Can you work these out from the model? Positions are in its coordinate system, mm. A direction names the side the tool comes from. Give positions to 0.01 mm unless a question says otherwise; leave off trailing zeros. Write each loop counter-clockwise with the first axis right and the second up, starting at its lowest first coordinate (ties: lowest second). Pieces come first, ordered by that corner, then holes.
from build123d import *

# Parameters (mm, degrees)
SKETCH1_R            = 50
BOSS_EXTRUDE1_DEPTH  = 5
SKETCH2_R            = 25.1
SKETCH2_R_2          = 21.1
SKETCH2_R_3          = 12.4
SKETCH2_R_4          = 9.399999999999999
BOSS_EXTRUDE2_DEPTH  = 5
CHAMFER1_SIZE        = 1
CUT_EXTRUDE1_START   = -5
SKETCH3_R            = 9.399999999999997
CUT_EXTRUDE1_DEPTH   = 5
CUT_EXTRUDE2_DEPTH   = 5
BOSS_EXTRUDE3_DEPTH  = 5
SKETCH6_R            = 1.5000000000000009
SKETCH6_R_2          = 1.5000000000000018
SKETCH6_R_3          = 1.500000000000004
SKETCH6_R_4          = 1.5000000000000042
CUT_EXTRUDE3_DEPTH   = 10
CUT_EXTRUDE4_DEPTH   = 4
CHAMFER4_SIZE        = 2
SKETCH10_R           = 21.638560794932243
SKETCH10_R_2         = 12.399999999999999
BOSS_EXTRUDE4_DEPTH  = 2
CHAMFER5_SIZE        = 5
SKETCH14_R           = 9.399999999999995
SKETCH14_R_2         = 3
BOSS_EXTRUDE6_DEPTH  = 10
SKETCH16_R           = 9.4
CUT_EXTRUDE8_DEPTH   = 4
FILLET3_R            = 4
BOSS_EXTRUDE7_START  = 30
BOSS_EXTRUDE7_DEPTH  = 30
SKETCH22_W           = 12
SKETCH22_H           = 13.999999999999996
BOSS_EXTRUDE10_DEPTH = 3
SKETCH23_R           = 1.0000000000000018
CUT_EXTRUDE11_DEPTH  = 3
BOSS_EXTRUDE11_DEPTH = 4


with BuildPart() as part:
    # Sketch1 → Boss-Extrude1 (new body)
    with BuildSketch(Plane(origin=(0, 0, 0), x_dir=(1, 0, 0), z_dir=(0, 1, 0))):
        with BuildLine():
            ThreePointArc((-43.30127018922194, -24.999999999999986), (-50, 6.12e-15), (-43.30127018922194, 24.999999999999996))
            Line((-43.301270189221945, 24.99999999999999), (-73.30127018922194, 25.000000000000004))
            Line((-73.30127018922194, 25.000000000000004), (-73.30127018922195, -24.999999999999996))
            Line((-73.30127018922195, -24.999999999999996), (-43.30127018922194, -24.99999999999999))
        make_face()
        Circle(SKETCH1_R)
    extrude(amount=BOSS_EXTRUDE1_DEPTH)

    # Sketch2 → Boss-Extrude2 (add)
    # profile 1 of 2: a face of its own
    with BuildSketch(Plane(origin=(0, 5, 0), x_dir=(1, 0, 0), z_dir=(0, 1, 0))):
        with Locations(Location((0, 0, 0), (0, 0, 270))):
            Circle(SKETCH2_R)
        with Locations(Location((0, 0, 0), (0, 0, 270))):
            Circle(SKETCH2_R_2, mode=Mode.SUBTRACT)
    # profile 2 of 2: a face of its own
    with BuildSketch(Plane(origin=(0, 5, 0), x_dir=(1, 0, 0), z_dir=(0, 1, 0))):
        with Locations(Location((0, 0, 0), (0, 0, 270))):
            Circle(SKETCH2_R_3)
        with Locations(Location((0, 0, 0), (0, 0, 270))):
            Circle(SKETCH2_R_4, mode=Mode.SUBTRACT)
    extrude(amount=BOSS_EXTRUDE2_DEPTH)

    # Chamfer1
    chamfer1_edges = [part.edges().sort_by_distance(p)[0] for p in [
        (3.8e-15, 10, -12.4),
    ]]
    chamfer(chamfer1_edges, length=CHAMFER1_SIZE)

    # Sketch3 → Cut-Extrude1 (cut)
    with BuildSketch(Plane(origin=(0, 5, 0), x_dir=(1, 0, 0), z_dir=(0, 1, 0)).offset(CUT_EXTRUDE1_START)):
        with Locations(Location((0, 0, 0), (0, 0, 270))):
            Circle(SKETCH3_R)
    extrude(amount=CUT_EXTRUDE1_DEPTH, mode=Mode.SUBTRACT)

    # Sketch4 → Cut-Extrude2 (cut)
    with BuildSketch(Plane(origin=(0, 5, 0), x_dir=(1, 0, 0), z_dir=(0, 1, 0))):
        with BuildLine():
            Line((-65.60000000000008, 17.09999999999999), (-58.60000000000002, 17.099999999999994))
            ThreePointArc((-58.60000000000002, 17.099999999999994), (-57.000000000000014, 15.499999999999982), (-58.60000000000005, 13.899999999999999))
            Line((-58.60000000000005, 13.899999999999999), (-65.60000000000005, 13.899999999999995))
            ThreePointArc((-65.60000000000005, 13.899999999999995), (-67.20000000000007, 15.49999999999998), (-65.60000000000008, 17.09999999999999))
        make_face()
        with BuildLine():
            Line((-34.600000000000044, 17.099999999999998), (-27.599999999999948, 17.099999999999998))
            ThreePointArc((-27.599999999999948, 17.099999999999998), (-25.999999999999968, 15.499999999999998), (-27.59999999999995, 13.899999999999999))
            Line((-27.59999999999995, 13.899999999999999), (-34.600000000000044, 13.899999999999999))
            ThreePointArc((-34.600000000000044, 13.899999999999999), (-36.20000000000004, 15.499999999999998), (-34.600000000000044, 17.099999999999998))
        make_face()
        with BuildLine():
            Line((-34.600000000000044, -17.1), (-27.599999999999945, -17.099999999999998))
            ThreePointArc((-27.599999999999945, -17.099999999999998), (-25.999999999999964, -15.5), (-27.599999999999945, -13.899999999999997))
            Line((-27.599999999999945, -13.899999999999997), (-34.600000000000044, -13.899999999999999))
            ThreePointArc((-34.600000000000044, -13.899999999999999), (-36.20000000000003, -15.500000000000002), (-34.600000000000044, -17.1))
        make_face()
        with BuildLine():
            Line((-65.60000000000005, -17.1), (-58.600000000000016, -17.1))
            ThreePointArc((-58.600000000000016, -17.1), (-56.999999999999986, -15.500000000000005), (-58.600000000000016, -13.900000000000006))
            Line((-58.600000000000016, -13.900000000000006), (-65.60000000000005, -13.900000000000006))
            ThreePointArc((-65.60000000000005, -13.900000000000006), (-67.20000000000007, -15.500000000000005), (-65.60000000000005, -17.1))
        make_face()
        with BuildLine():
            Line((-58.10000000000014, 11.500000000000004), (-35.10000000000015, 11.500000000000004))
            ThreePointArc((-35.10000000000015, 11.500000000000004), (-30.336544032709547, -8.3e-16), (-35.10000000000015, -11.500000000000004))
            Line((-35.10000000000015, -11.500000000000004), (-58.10000000000014, -11.50000000000001))
            ThreePointArc((-58.10000000000014, -11.50000000000001), (-62.863455967290705, -6.4e-16), (-58.10000000000014, 11.500000000000004))
        make_face()
    extrude(amount=-CUT_EXTRUDE2_DEPTH, mode=Mode.SUBTRACT)

    # Sketch5 → Boss-Extrude3 (add)
    with BuildSketch(Plane(origin=(0, 5, 0), x_dir=(1, 0, 0), z_dir=(0, 1, 0))):
        with BuildLine():
            ThreePointArc((-43.30127018922194, -24.99999999999999), (50, 2.22e-14), (-43.301270189221945, 24.99999999999998))
            ThreePointArc((-43.301270189221945, 24.99999999999998), (-29.51879380479877, 25.25375244111435), (-19.593681219974982, 15.68749999999999))
            ThreePointArc((-19.593681219974982, 15.68749999999999), (25.099999999999998, 0), (-19.593681219974982, -15.68749999999999))
            ThreePointArc((-19.593681219974982, -15.68749999999999), (-29.518793804798747, -25.253752441114404), (-43.30127018922194, -24.99999999999999))
        make_face()
    extrude(amount=BOSS_EXTRUDE3_DEPTH)

    # Sketch6 → Cut-Extrude3 (cut)
    with BuildSketch(Plane(origin=(0, 10, 0), x_dir=(1, 0, 0), z_dir=(0, 1, 0))):
        with Locations(Location((8.000000000000004, -35.55, 0), (0, 0, 270))):
            Circle(SKETCH6_R)
        with Locations(Location((-8, -35.55, 0), (0, 0, 90))):
            Circle(SKETCH6_R_2)
        with Locations(Location((8.000000000000004, 35.55, 0), (0, 0, 90))):
            Circle(SKETCH6_R)
        with Locations(Location((-8, 35.55, 0), (0, 0, 270))):
            Circle(SKETCH6_R_2)
        with Locations(Location((35.55, -8, 0), (0, 0, 270))):
            Circle(SKETCH6_R_3)
        with Locations(Location((35.55, 8, 0), (0, 0, 90))):
            Circle(SKETCH6_R_4)
    extrude(amount=-CUT_EXTRUDE3_DEPTH, mode=Mode.SUBTRACT)

    # Sketch7 → Cut-Extrude4 (cut)
    with BuildSketch(Plane(origin=(0, 10, 0), x_dir=(1, 0, 0), z_dir=(0, 1, 0))):
        Polygon((-7.9999999999999964, -38.650000000000006), (-5.315321248268234, -37.1), (-5.315321248268235, -34), (-7.9999999999999964, -32.45000000000001), (-10.684678751731763, -34.00000000000001), (-10.684678751731763, -37.1), align=None)
        Polygon((8.000000000000005, -38.650000000000006), (10.684678751731774, -37.099999999999994), (10.684678751731772, -33.999999999999986), (8.00000000000001, -32.449999999999996), (5.315321248268237, -34), (5.315321248268238, -37.099999999999994), align=None)
        Polygon((5.315321248268238, 37.099999999999994), (8.000000000000005, 38.650000000000006), (10.684678751731774, 37.099999999999994), (10.684678751731772, 33.999999999999986), (8.00000000000001, 32.449999999999996), (5.315321248268237, 34), align=None)
        Polygon((-10.684678751731763, 37.1), (-7.9999999999999964, 38.650000000000006), (-5.315321248268234, 37.1), (-5.315321248268235, 34), (-7.9999999999999964, 32.45000000000001), (-10.684678751731763, 34.00000000000001), align=None)
        Polygon((32.68508267298749, 6.815834171501503), (35.1430590262669, 4.926825900815709), (38.00797635327939, 6.110991729314209), (38.4149173270125, 9.184165828498493), (35.956940973733104, 11.073174099184284), (33.0920236467206, 9.88900827068578), align=None)
        Polygon((32.68365214703024, -9.180698939516597), (35.13934134935783, -11.072679526513099), (38.005689202327595, -9.891980586996501), (38.416347852969764, -6.819301060483406), (35.96065865064216, -4.927320473486905), (33.0943107976724, -6.108019413003499), align=None)
    extrude(amount=-CUT_EXTRUDE4_DEPTH, mode=Mode.SUBTRACT)

    # Chamfer4
    chamfer4_edges = [part.edges().sort_by_distance(p)[0] for p in [
        (-25.1, 10, -9.22e-15),
    ]]
    chamfer(chamfer4_edges, length=CHAMFER4_SIZE)

    # Sketch10 → Boss-Extrude4 (add)
    with BuildSketch(Plane(origin=(0, 5, 0), x_dir=(1, 0, 0), z_dir=(0, 1, 0))):
        Circle(SKETCH10_R)
        with Locations(Location((0, 0, 0), (0, 0, 270))):
            Circle(SKETCH10_R_2, mode=Mode.SUBTRACT)
    extrude(amount=BOSS_EXTRUDE4_DEPTH)

    # Chamfer5
    chamfer5_edges = [part.edges().sort_by_distance(p)[0] for p in [
        (50.00000000000001, 10, -2.487e-14),
    ]]
    chamfer(chamfer5_edges, length=CHAMFER5_SIZE)

    # Sketch14 → Boss-Extrude6 (add)
    with BuildSketch(Plane.XZ):
        Circle(SKETCH14_R)
        with Locations(Location((0, 0, 0), (0, 0, 90))):
            Circle(SKETCH14_R_2, mode=Mode.SUBTRACT)
    extrude(amount=-BOSS_EXTRUDE6_DEPTH)

    # Sketch16 → Cut-Extrude8 (cut)
    with BuildSketch(Plane.XZ):
        with Locations(Location((0, 0, 0), (0, 0, 270))):
            Circle(SKETCH16_R)
    extrude(amount=-CUT_EXTRUDE8_DEPTH, mode=Mode.SUBTRACT)

    # Fillet3
    fillet3_edges = [part.edges().sort_by_distance(p)[0] for p in [
        (-73.30127018922195, 2.5, 24.999999999999996),
        (-73.30127018922194, 2.5, -25.000000000000004),
    ]]
    fillet(fillet3_edges, radius=FILLET3_R)

    # Sketch17 → Boss-Extrude7 (add)
    with BuildSketch(Plane(origin=(0, 5, 0), x_dir=(1, 0, 0), z_dir=(0, 1, 0)).offset(BOSS_EXTRUDE7_START)):
        with BuildLine():
            Line((-65.30127018922194, 24.999999999999968), (-65.30127018922194, 21.000000000000004))
            Line((-65.30127018922194, 21.000000000000004), (-73.30127018922195, 21))
            ThreePointArc((-73.30127018922195, 21), (-72.12969731396817, 23.82842712474621), (-69.30127018922194, 24.999999999999968))
            Line((-69.30127018922194, 24.999999999999968), (-65.30127018922194, 24.999999999999968))
        make_face()
    extrude(amount=-BOSS_EXTRUDE7_DEPTH)

    # Sketch22 → Boss-Extrude10 (add)
    with BuildSketch(Plane(origin=(-65.30127018922194, 0, 0), x_dir=(0, 0, -1), z_dir=(1, 0, 0))):
        with Locations((18.999999999999964, 27.999999999999993)):
            Rectangle(SKETCH22_W, SKETCH22_H)
    extrude(amount=BOSS_EXTRUDE10_DEPTH)

    # Sketch23 → Cut-Extrude11 (cut)
    with BuildSketch(Plane.ZY.offset(65.30127018922194)):
        with Locations((-17.999999999999968, 31.599999999999998)):
            Circle(SKETCH23_R)
        with Locations((-17.999999999999968, 25.089999999999993)):
            Circle(SKETCH23_R)
    extrude(amount=-CUT_EXTRUDE11_DEPTH, mode=Mode.SUBTRACT)

    # Sketch24 → Boss-Extrude11 (add)
    with BuildSketch(Plane(origin=(1.156e-14, 0, -24.99999999999997), x_dir=(-1, 0, -4.6e-16), z_dir=(4.6e-16, 0, -1))):
        Polygon((62.30127018922195, 20.999999999999996), (62.30127018922195, 5.000000000000001), (65.30127018922195, 5), (65.30127018922195, 20.999999999999996), align=None)
    extrude(amount=-BOSS_EXTRUDE11_DEPTH)


solid = part.part
(1) If I drill on L1, parallel to Y at x = -64, z = -18; L2, parallel to X at y = 1.9, z = -8; L3, parallel to X at y = 2, z = -5, over which ranges is the centre line in solid material (lowest first)?
Returned:
L1: y = 0 to 5, 21 to 24.09, 26.09 to 30.6, 32.6 to 35
L2: x = -73.3 to -60.76, -32.44 to -4.94, 4.94 to 34.05, 37.05 to 49.36
L3: x = -73.3 to -62.08, -31.12 to -7.96, 7.96 to 49.75
(2) For faces 1 (the face through (-23.224, 9.875, -0.22)), 2 (the face through (-73.301, 2, 0)), 3 (the face through (-47, 3, -11.5)), 4 (the face through (2.824, 1.972, -8.966)), 5 (the face through (-6.7, 8, 37.9)), which set-ups out of +Z, -Z, +X, -X, +Y, -Y let a thin tool reach every point of the face, with its end or its side?
Returned:
face 1: -X, +Y
face 2: +Z, -Z, -X, +Y, -Y
face 3: +Y, -Y
face 4: -Y
face 5: +Y
(3) If we mould it in two halves opening along Z, with no side actions, what happens to faces 6 (the face through (-31, 3, 13.9)), 7 (the face through (-9.3, 8, 33.2)), 8 (the face through (-62.301, 24, -20))? For each: +Z half, -Z half, draft (parallel to the pull), parting line (faces both ways), or undercut.
Returned:
face 6: undercut
face 7: undercut
face 8: draft
(4) Imagine slicing it at C-C, the plane y = 29. Write out the boundary of the cut face in (x, z), plus the area to 3 significant figures.
Returned:
outline: (-73.3, -21) arc R4 ccw to (-69.3, -25) - (-62.3, -25) - (-62.3, -13) - (-65.3, -13) - (-65.3, -21) - close
area: 64.6 mm2
(5) Will these pins go through, and if not, where does the flat tip stop? P1, Ø5.5, axis at x = -43, y = 2.5, coming from the +Z side; P2, Ø5, axis at x = 8, z = 35.55, coming from the +Y side; P3, Ø8, axis at y = 9.5, z = 5.5, coming from the +X side; P4, Ø2.5, axis at x = 35.55, z = 8, coming from the +Y side.
Returned:
P1: stops at z = 29.66
P2: stops at y = 6
P3: stops at x = 49.22
P4: passes through
(6) Imagine slicing it at B-B, the plane x = 0. Write out the boundary of the cut face in (y, z).
Returned:
outline: (0, -50) - (5, -50) - (10, -45) - (10, -21.1) - (7, -21.1) - (7, -12.4) - (9, -12.4) - (10, -11.4) - (10, -3) - (4, -3) - (4, -9.4) - (0, -9.4) - close; (0, 9.4) - (4, 9.4) - (4, 3) - (10, 3) - (10, 11.4) - (9, 12.4) - (7, 12.4) - (7, 21.1) - (10, 21.1) - (10, 45) - (5, 50) - (0, 50) - close
(7) Imagine slicing it at D-D, the plane x = -48. Write out the boundary of the cut face in (y, z), plus the area to 3 significant figures.
Returned:
outline: (0, -25) - (5, -25) - (5, -11.5) - (0, -11.5) - close; (0, 11.5) - (5, 11.5) - (5, 25) - (0, 25) - close
area: 135 mm2
(8) Imagine slicing it at A-A, the plane z = 0. Give the number of separate pieces and of enclosed holes in the cut face, plus the area to 3 significant figures.
Returned:
separate pieces: 3
enclosed holes: 0
area: 650 mm2
